For this review, take the finished solid that the model builds, in its own axes (mm). A direction names the side the tool comes from. Round coordinates to 2 decimals unless told otherwise and drop trailing zeros. Order: outer loops, then holes, each group sorted by start corner. A loop starts at its lowest first (then second) coordinate and runs counter-clockwise, first axis right, second up. Notation, with made-up numbers: (89.5, 77.25) -> (147.5, 77.25) arc R22 cw to (147.5, 85.25) -> close; hole circle Ø2 at (7.5, 73.25). An arc over 180 degrees is marked (long way). Answer in a Markdown table with one row per item.
```python
from build123d import *

# Parameters (mm, degrees)
SKETCH1_W           = 90
SKETCH1_H           = 100
BOSS_EXTRUDE1_DEPTH = 2
BOSS_EXTRUDE2_DEPTH = 8
SKETCH3_W           = 4
SKETCH3_H           = 4
CUT_EXTRUDE2_DEPTH  = 3


with BuildPart() as part:
    # Sketch1 → Boss-Extrude1 (new body)
    with BuildSketch(Plane.XY):
        Rectangle(SKETCH1_W, SKETCH1_H)
    extrude(amount=-BOSS_EXTRUDE1_DEPTH)

    # Sketch2 → Boss-Extrude2 (add)
    with BuildSketch(Plane(origin=(0, 0, -2), x_dir=(-1, 0, 0), z_dir=(0, 0, -1))):
        Polygon((-45, 50), (-45, -50), (-40, -50), (-40, -47.5), (-40, 45), (40, 45), (40, -47.5), (40, -50), (45, -50), (45, 50), align=None)
    extrude(amount=BOSS_EXTRUDE2_DEPTH)

    # Sketch3 → Cut-Extrude2 (cut)
    with BuildSketch(Plane(origin=(0, 0, -10), x_dir=(-1, 0, 0), z_dir=(0, 0, -1))):
        with Locations((-42.5, 47.5)):
            Rectangle(SKETCH3_W, SKETCH3_H)
        with Locations((42.5, 47.5)):
            Rectangle(SKETCH3_W, SKETCH3_H)
        with Locations((42.5, -47.5)):
            Rectangle(SKETCH3_W, SKETCH3_H)
        with Locations((-42.5, -47.5)):
            Rectangle(SKETCH3_W, SKETCH3_H)
    extrude(amount=-CUT_EXTRUDE2_DEPTH, mode=Mode.SUBTRACT)


solid = part.part
```
Q1. Tool access review of faces 1 (the face through (-40.5, 47, -9)), 2 (the face through (4, -50, -1)), 3 (the face through (40, -3, -6)): name each direction out of +Z, -Z, +X, -X, +Y, -Y from which nothing blocks a thin tool from reaching the whole face with its end or side.
Answer key:
| item | result |
|---|---|
| face 1 | -Z |
| face 2 | +Z, -Z, +X, -X, -Y |
| face 3 | -Z, -Y |
Q2. Take a section at A-A, the plane z = -5.5. Write out the cut boundary in (x, y).
Answer key:
| item | result |
|---|---|
| outline | (-45, -50) -> (-40, -50) -> (-40, 45) -> (40, 45) -> (40, -50) -> (45, -50) -> (45, 50) -> (-45, 50) -> close |
Q3. To check wall thickness, follow probe 1 along X at (y, z) = (12.5, -4.25); probe 2 along Y at (x, z) = (17, -6.25); probe 3 along Z at (x, y) = (-5, 25.5). State the ranges of each line that lie inside material, in increasing order.
Answer key:
| item | result |
|---|---|
| probe 1 | x = -45 to -40, 40 to 45 |
| probe 2 | y = 45 to 50 |
| probe 3 | z = -2 to 0 |
Q4. Take a section at B-B, the plane y = -23. Write out the cut boundary in (x, z).
Answer key:
| item | result |
|---|---|
| outline | (-45, -10) -> (-40, -10) -> (-40, -2) -> (40, -2) -> (40, -10) -> (45, -10) -> (45, 0) -> (-45, 0) -> close |
Q5. Clearance check with a flat-ended pin moving along its axis: pin 1 Ø1 at (x, y) = (10.5, -23) entering from -Z. State where the tip first meets the part, or that it passes through.
Answer key:
| item | result |
|---|---|
| pin 1 | stops at z = -2 |
Q6. Take a section at C-C, the plane x = 12. Write out the cut boundary in (y, z), then the cut area to 3 significant figures.
Answer key:
| item | result |
|---|---|
| outline | (-50, -2) -> (45, -2) -> (45, -10) -> (50, -10) -> (50, 0) -> (-50, 0) -> close |
| area | 240 mm^2 |
Q7. The part is to be moulded in two halves that separate along Y. For faces 4 (the face through (40.2, 11.3, -10)), 5 (the face through (43, 48, -7)), 6 (the face through (-1, 50, -5)), say which applies: +Y half, -Y half, draft (parallel to the pull), parting line (faces both ways), or undercut.
Answer key:
| item | result |
|---|---|
| face 4 | draft |
| face 5 | undercut |
| face 6 | +Y half |
